```python
from build123d import *

# Parameters (mm, degrees)
SKETCH1_W           = 5
SKETCH1_H           = 5
BOSS_EXTRUDE1_DEPTH = 2
SKETCH2_W           = 3.2
SKETCH2_H           = 3
BOSS_EXTRUDE2_DEPTH = 5
SKETCH3_W           = 3.2
SKETCH3_H           = 3.4
BOSS_EXTRUDE3_DEPTH = 3
CUT_EXTRUDE1_DEPTH  = 12.093241186


with BuildPart() as part:
    # Sketch1 → Boss-Extrude1 (new body)
    with BuildSketch(Plane(origin=(0, 0, 0), x_dir=(1, 0, 0), z_dir=(0, 1, 0))):
        Rectangle(SKETCH1_W, SKETCH1_H)
    extrude(amount=BOSS_EXTRUDE1_DEPTH)

    # Sketch2 → Boss-Extrude2 (add)
    with BuildSketch(Plane(origin=(0, 2, 0), x_dir=(1, 0, 0), z_dir=(0, 1, 0))):
        with Locations((0, 1)):
            Rectangle(SKETCH2_W, SKETCH2_H)
    extrude(amount=BOSS_EXTRUDE2_DEPTH)

    # Sketch3 → Boss-Extrude3 (add)
    with BuildSketch(Plane(origin=(0, 7, 0), x_dir=(1, 0, 0), z_dir=(0, 1, 0))):
        with Locations((0, 0.8)):
            Rectangle(SKETCH3_W, SKETCH3_H)
    extrude(amount=BOSS_EXTRUDE3_DEPTH)

    # Sketch4 → Cut-Extrude1 (cut, through all)
    with BuildSketch(Plane(origin=(1.6, 0, 0), x_dir=(0, 0, -1), z_dir=(1, 0, 0))):
        Polygon((-0.9, 7), (0.75, 10), (-0.9, 10), align=None)
    extrude(amount=-CUT_EXTRUDE1_DEPTH, mode=Mode.SUBTRACT)


solid = part.part
```
The listing builds one solid part. Answer for the finished solid, in the listing's coordinates (mm). A direction names the side the tool comes from. Give positions to 0.01 mm unless a question says otherwise; leave off trailing zeros. Write each loop counter-clockwise with the first axis right and the second up, starting at its lowest first coordinate (ties: lowest second). Pieces come first, ordered by that corner, then holes. Notation, with made-up numbers: (59.5, 53.5) -> (118.5, 53.5) arc R15 cw to (118.5, 75.5) -> close; hole circle Ø2 at (52, -14). An arc over 180 degrees is marked (long way). Write item = value, one per line. Start each with the question number.
1) The part is cut by section D-D, the plane z = 2.05. Determine the outline of the cut face in (x, y), and give its area (3 significant figures).
2) Each of these flat-tipped pins is pushed along its axis until it touches: pin 1 (2 mm diameter, centred on y = 6.5, z = -1.5, fed in from -X); pin 2 (1.5 mm diameter, centred on x = -1.5, z = 0.5, fed in from +Y); pin 3 (1 mm diameter, centred on y = 6.5, z = -1.5, fed in from +X). Where does it stop, or does it pass through?
3) The part is cut by section A-A, the plane x = -0.1. Determine the outline of the cut face in (y, z), and give its area (3 significant figures).
4) Straight lines are drawn through the part: line 1 along Y through (x, z) = (-0.05, 1.9); line 2 along Z through (x, y) = (1.2, 4.5); line 3 along X through (y, z) = (7.75, -1.1). For each, find the intervals that lie inside material, in ascending order.
5) Which of the six approach directions +Z, -Z, +X, -X, +Y, -Y give full straight-line access (tool end or side, diameter ignored) to faces 1 (the face through (-1.6, 6, -1)), 2 (the face through (0, 4, 0.5)), 3 (the face through (0, 4, -2.5)), 4 (the face through (1.6, 6, -1))?
6) The part is cut by section B-B, the plane z = 0.35. Determine the outline of the cut face in (x, y).
7) The part is cut by section C-C, the plane y = 3.5. Determine the outline of the cut face in (x, z), and give its area (3 significant figures).
Solutions:
q1.outline = (-2.5, 0) -> (2.5, 0) -> (2.5, 2) -> (-2.5, 2) -> close
q1.area = 10.0 mm²
q2.pin_1 = -1.6
q2.pin_2 = 9.09
q2.pin_3 = 1.6
q3.outline = (0, -2.5) -> (10, -2.5) -> (10, -0.75) -> (7, 0.9) -> (7, 0.5) -> (2, 0.5) -> (2, 2.5) -> (0, 2.5) -> close
q3.area = 32.7 mm²
q4.line_1 = 0 to 2
q4.line_2 = -2.5 to 0.5
q4.line_3 = -1.6 to 1.6
q5.face_1 = +Z, -Z, -X, +Y
q5.face_2 = +Z, +X, -X
q5.face_3 = -Z, +X, -X, +Y, -Y
q5.face_4 = +Z, -Z, +X, +Y
q6.outline = (-2.5, 0) -> (2.5, 0) -> (2.5, 2) -> (1.6, 2) -> (1.6, 8) -> (-1.6, 8) -> (-1.6, 2) -> (-2.5, 2) -> close
q7.outline = (-1.6, -2.5) -> (1.6, -2.5) -> (1.6, 0.5) -> (-1.6, 0.5) -> close
q7.area = 9.60 mm²
